CAD build for the part. Positions are in the model's coordinates, mm. Face numbers are marked on the shaded views. A direction names the side the tool comes from. Round coordinates to 2 decimals unless told otherwise and drop trailing zeros. Order: outer loops, then holes, each group sorted by start corner. A loop starts at its lowest first (then second) coordinate and runs counter-clockwise, first axis right, second up. Notation, with made-up numbers: (6.25, 81) - (33.25, 81) arc R19 cw to (33.25, 100) - close; hole circle Ø7 at (34.5, 31.25). An arc over 180 degrees is marked (long way). Write item = value, one per line.
from build123d import *

# Parameters (mm, degrees)
SKETCH1_W           = 11.9634
SKETCH1_H           = 9.9568
BOSS_EXTRUDE1_DEPTH = 9.017
BOSS_EXTRUDE2_DEPTH = 10.0584
SKETCH3_R           = 1.9939
BOSS_EXTRUDE3_DEPTH = 0.762
BOSS_EXTRUDE4_DEPTH = 16.51


with BuildPart() as part:
    # Sketch1 → Boss-Extrude1 (new body)
    with BuildSketch(Plane(origin=(0, 0, 0), x_dir=(0, 0, -1), z_dir=(1, 0, 0))):
        Rectangle(SKETCH1_W, SKETCH1_H)
    extrude(amount=-BOSS_EXTRUDE1_DEPTH)

    # Sketch2 → Boss-Extrude2 (add)
    with BuildSketch(Plane(origin=(0, 0, 0), x_dir=(0, 0, -1), z_dir=(1, 0, 0))):
        with BuildLine():
            Line((-1.101610621, 1.016), (1.101610621, 1.016))
            ThreePointArc((1.101610621, 1.016), (0, -1.4986), (-1.101610621, 1.016))
        make_face()
    extrude(amount=BOSS_EXTRUDE2_DEPTH)

    # Sketch3 → Boss-Extrude3 (add)
    with BuildSketch(Plane(origin=(0, 0, 0), x_dir=(0, 0, -1), z_dir=(1, 0, 0))):
        Circle(SKETCH3_R)
    extrude(amount=BOSS_EXTRUDE3_DEPTH)

    # Sketch4 → Boss-Extrude4 (add)
    with BuildSketch(Plane.ZY.offset(9.017)):
        with BuildLine():
            Line((-3.406844536, 4.9784), (3.406844536, 4.9784))
            ThreePointArc((3.406844536, 4.9784), (6.0325, 0), (3.406844536, -4.9784))
            Line((3.406844536, -4.9784), (-3.406844536, -4.9784))
            ThreePointArc((-3.406844536, -4.9784), (-6.0325, 0), (-3.406844536, 4.9784))
        make_face()
    extrude(amount=BOSS_EXTRUDE4_DEPTH)


solid = part.part
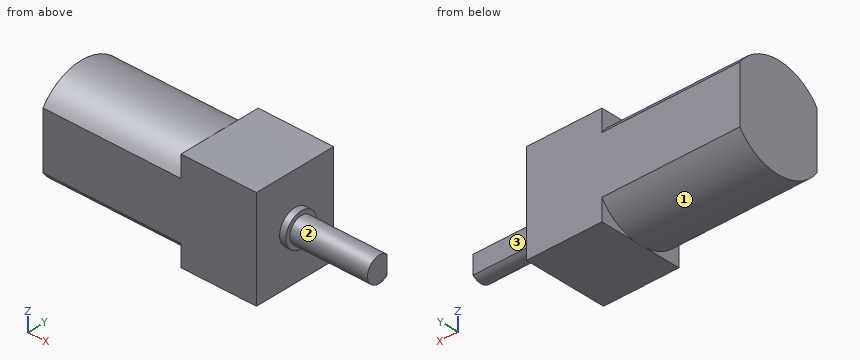
(1) Drop flat-ended pins along their axis: pin 1 (2.5 mm diameter, centred on x = -6.5, y = -0.5, fed in from -Z); pin 2 (2.5 mm diameter, centred on x = 3.5, z = 0.5, fed in from +Y); pin 3 (3 mm diameter, centred on y = -2.5, z = 0, fed in from +X). Give the stop position or say it passes through.
Solved:
pin_1 = -5.98
pin_2 = 1.02
pin_3 = 10.06
(2) Band-saw the part on D-D on y = 2.5. List the corners of the cut face in (x, z).
Solved:
outline = (-25.53, -5.49) - (-9.02, -5.49) - (-9.02, -5.98) - (0, -5.98) - (0, 5.98) - (-9.02, 5.98) - (-9.02, 5.49) - (-25.53, 5.49) - close
(3) Tool access for the marked faces 1, 2 and 3: list every direction of +Z, -Z, +X, -X, +Y, -Y with a clear straight run to the whole face (end or side of a thin tool).
Solved:
face_1 = -Z, -X
face_2 = +X
face_3 = +Z, -Z, +X, +Y
(4) Band-saw the part on C-C on x = 5.5. List the corners of the cut face in (y, z), plus the area to 3 significant figures.
Solved:
outline = (1.02, -1.1) - (1.02, 1.1) arc R1.5 ccw (long way) to start
area = 6.32 mm²
(5) Probe line 1 along X through (y, z) = (-3.5, 4.5); line 2 along Z through (x, y) = (-4, -0.5); line 3 along Y through (x, z) = (4.5, 0). List the from-to ranges inside material, lowest first.
Solved:
line_1 = -25.53 to 0
line_2 = -5.98 to 5.98
line_3 = -1.5 to 1.02
(6) Band-saw the part on A-A on y = 0. List the corners of the cut face in (x, z).
Solved:
outline = (-25.53, -6.03) - (-9.02, -6.03) - (-9.02, -5.98) - (0, -5.98) - (0, -1.99) - (0.76, -1.99) - (0.76, -1.5) - (10.06, -1.5) - (10.06, 1.5) - (0.76, 1.5) - (0.76, 1.99) - (0, 1.99) - (0, 5.98) - (-9.02, 5.98) - (-9.02, 6.03) - (-25.53, 6.03) - close
(7) Band-saw the part on B-B on z = 0. List the corners of the cut face in (x, y).
Solved:
outline = (-25.53, -4.98) - (0, -4.98) - (0, -1.99) - (0.76, -1.99) - (0.76, -1.5) - (10.06, -1.5) - (10.06, 1.02) - (0.76, 1.02) - (0.76, 1.99) - (0, 1.99) - (0, 4.98) - (-25.53, 4.98) - close
